```python
from build123d import *

# Parameters (mm, degrees)
EXTRUDE_THIN1_DEPTH = 222.25
FILLET1_R           = 1.016


with BuildPart() as part:
    # Sketch1 → Extrude-Thin1 (new body)
    with BuildSketch(Plane.XY):
        with BuildLine():
            Line((0, 0), (0, -9.525))
            Line((0, -9.525), (-3.175, -9.525))
            Line((-3.175, -9.525), (-3.175, -6.693600755))
            ThreePointArc((-3.175, -6.693600755), (-4.128572785, -4.828192758), (-4.7625, -2.831399245))
            Line((-4.7625, -2.831399245), (-4.7625, 0))
            Line((-4.7625, 0), (-6.35, 0))
            Line((-6.35, 0), (-6.35, 12.7))
            Line((-6.35, 12.7), (9.525, 12.7))
            Line((9.525, 12.7), (9.525, 11.684))
            Line((9.525, 11.684), (-5.334, 11.684))
            Line((-5.334, 11.684), (-5.334, 1.016))
            Line((-5.334, 1.016), (-3.7465, 1.016))
            Line((-3.7465, 1.016), (-3.7465, -2.714277453))
            ThreePointArc((-3.7465, -2.714277453), (-3.111980098, -4.624554555), (-2.159, -6.397575437))
            Line((-2.159, -6.397575437), (-2.159, -8.509))
            Line((-2.159, -8.509), (-1.016, -8.509))
            Line((-1.016, -8.509), (-1.016, 0))
            Line((-1.016, 0), (0, 0))
        make_face()
    extrude(amount=-EXTRUDE_THIN1_DEPTH)

    # Fillet1
    fillet1_edges = [part.edges().sort_by_distance(p)[0] for p in [
        (-3.7465, 1.016, -111.125),
        (-2.159, -6.397575437, -111.125),
        (0, -9.525, -111.125),
        (-3.175, -9.525, -111.125),
        (-4.7625, -2.831399245, -111.125),
        (-6.35, 0, -111.125),
        (-6.35, 12.7, -111.125),
    ]]
    fillet(fillet1_edges, radius=FILLET1_R)


solid = part.part
```
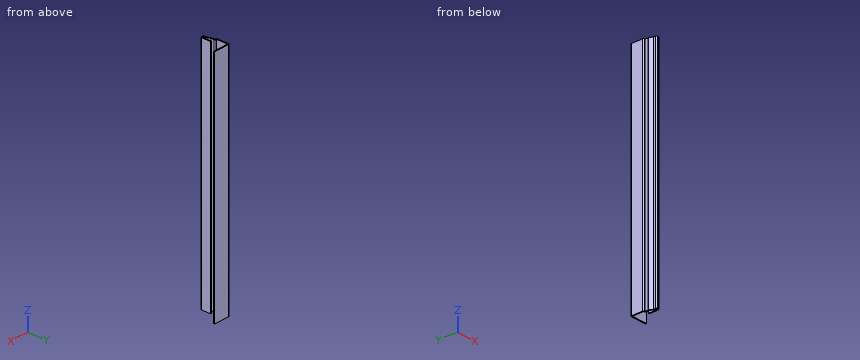
Verification items for the finished model (mm, model axes). Round coordinates to 2 decimals unless told otherwise and drop trailing zeros. Order: outer loops, then holes, each group sorted by start corner. A loop starts at its lowest first (then second) coordinate and runs counter-clockwise, first axis right, second up. Notation, with made-up numbers: (75, 69.5) - (104, 69.5) arc R19 ccw to (104, 91.5) - close; hole circle Ø2 at (39, 17). An arc over 180 degrees is marked (long way). Use CSV: the item, a comma, the result in double quotes. Start each with the question number.
1) Section check B-B, the plane x = 5. Record the cut outline in (y, z).
2) Thickness scan on L1, parallel to Y at x = -0.75, z = -25; L2, parallel to X at y = -2, z = -86; L3, parallel to Y at x = -1.25, z = -180.5 (3 decimals). Record the ranges inside material, lowest first.
3) Go/stop test with flat-tipped pins: P1, Ø4, axis at x = 5.5, z = -61, coming from the -Y side; P2, Ø3, axis at y = -1, z = -102.5, coming from the +X side; P3, Ø3, axis at y = -1, z = -126.5, coming from the -X side; P4, Ø1.5, axis at x = 2, y = -0.5, coming from the +Z side. Record where each tip stops, or that it passes through.
4) Section check C-C, the plane y = 4. Record the cut outline in (x, z).
Answers:
1,outline,"(11.68, -222.25) - (12.7, -222.25) - (12.7, 0) - (11.68, 0) - close"
2,L1,"y = -9.49 to 0, 11.68 to 12.7"
2,L2,"x = -4.76 to -3.75, -1.02 to 0"
2,L3,"y = -9.525 to -8.509, 11.684 to 12.7"
3,P1,"stops at y = 11.68"
3,P2,"stops at x = 0"
3,P3,"stops at x = -6.21"
3,P4,"passes through"
4,outline,"(-6.35, -222.25) - (-5.33, -222.25) - (-5.33, 0) - (-6.35, 0) - close"
